```python
from build123d import *

# Parameters (mm, degrees)
SKETCH2_R           = 2.95
BOSS_EXTRUDE1_DEPTH = 9
SKETCH3_W           = 2.54
SKETCH3_H           = 0.5
BOSS_EXTRUDE2_DEPTH = 5


with BuildPart() as part:
    # Sketch2 → Boss-Extrude1 (new body)
    with BuildSketch(Plane(origin=(0, 0, 0), x_dir=(1, 0, 0), z_dir=(0, 1, 0))):
        with Locations(Location((0, 0, 0), (0, 0, 270))):
            Circle(SKETCH2_R)
    extrude(amount=BOSS_EXTRUDE1_DEPTH)

    # Sketch3 → Boss-Extrude2 (add)
    with BuildSketch(Plane.XZ):
        Rectangle(SKETCH3_W, SKETCH3_H)
    extrude(amount=BOSS_EXTRUDE2_DEPTH)


solid = part.part
```
Part model, mm, in its own coordinate system. A direction names the side the tool comes from. Round coordinates to 2 decimals unless told otherwise and drop trailing zeros. Loops run counter-clockwise (first coordinate to the right, second up) from the corner with the lowest first, then second, coordinate; pieces in that order, holes last.
Item 1: Cut at C-C, the plane y = 6. Give the cut face in (x, z), then the cut area to 3 significant figures.
Item 2: Cut at A-A, the plane x = 0. Give the cut face in (y, z).
Item 3: Cut at D-D, the plane y = -3.25. Give the cut face in (x, z).
Item 4: Drill centre lines: line 1 (Y direction, x = -0.5, z = -0.75); line 2 (Z direction, x = 0.5, y = -2.75); line 3 (X direction, y = -1.5, z = -0.05). Where is each one in solid material? Low to high.
Item 5: 3-axis set-ups, long thin cutter, end or side, ignore diameter. For faces 1 (the face through (0, -2, 0.25)), 2 (the face through (-2.88, 4.44, -0.64)), 3 (the face through (0, -2, -0.25)): which of +Z, -Z, +X, -X, +Y, -Y reach the whole face in a straight line?
Item 6: Drop flat-ended pins along their axis: P1, Ø1.3, axis at x = -0.5, y = -2, coming from the -Z side; P2, Ø3, axis at x = -1.5, z = 2, coming from the -Y side; P3, Ø1.3, axis at x = -0.5, y = -3.5, coming from the +Z side. Give the stop position or say it passes through.
Item 7: Cut at B-B, the plane z = 0. Give the cut face in (x, y).
A:
1. outline: circle Ø5.9 at (0, 0)
1. area: 27.3 mm2
2. outline: (-5, -0.25) - (0, -0.25) - (0, -2.95) - (9, -2.95) - (9, 2.95) - (0, 2.95) - (0, 0.25) - (-5, 0.25) - close
3. outline: (-1.27, -0.25) - (1.27, -0.25) - (1.27, 0.25) - (-1.27, 0.25) - close
4. line 1: y = 0 to 9
4. line 2: z = -0.25 to 0.25
4. line 3: x = -1.27 to 1.27
5. face 1: +Z, +X, -X, -Y
5. face 2: +Y, -Y
5. face 3: -Z, +X, -X, -Y
6. P1: stops at z = -0.25
6. P2: stops at y = 0
6. P3: stops at z = 0.25
7. outline: (-2.95, 0) - (-1.27, 0) - (-1.27, -5) - (1.27, -5) - (1.27, 0) - (2.95, 0) - (2.95, 9) - (-2.95, 9) - close
